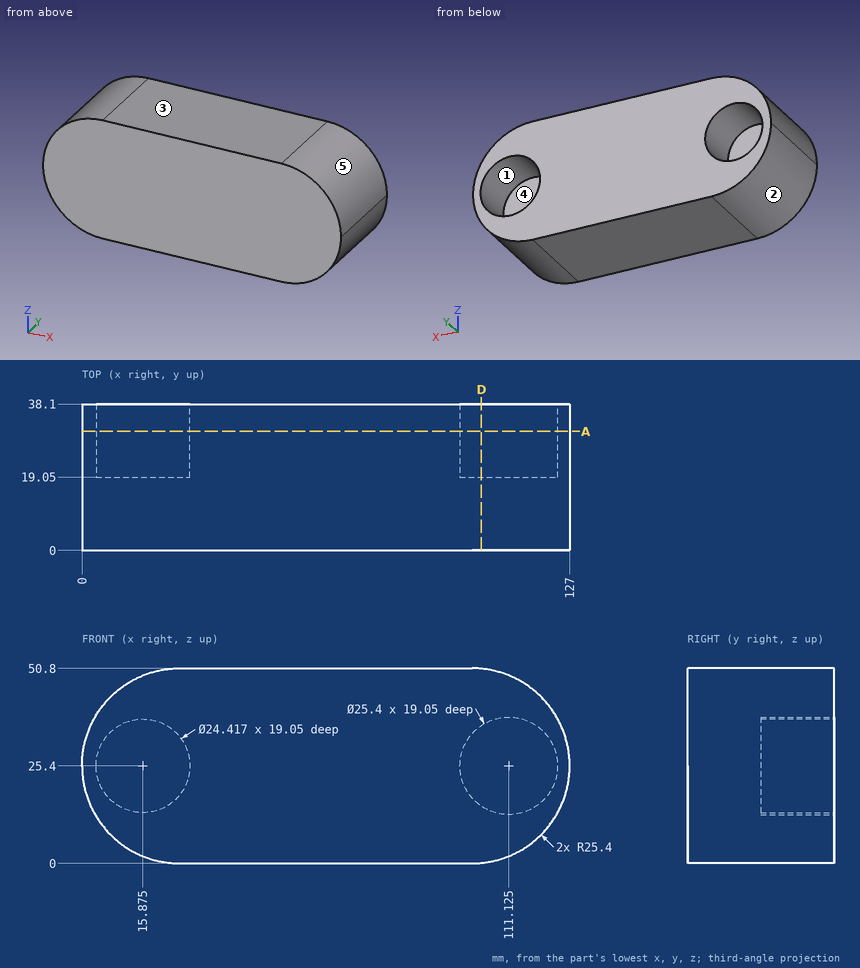
Source: three-view drawing plus pictorial views. Frame: mm from the lowest corner of the part. A direction names the side the tool comes from. Give positions to 0.01 mm unless a question says otherwise; leave off trailing zeros. Write each loop counter-clockwise with the first axis right and the second up, starting at its lowest first coordinate (ties: lowest second). Pieces come first, ordered by that corner, then holes. Notation, with made-up numbers: (12.5, -34.5) - (52.5, -34.5) arc R22 cw to (52.5, -18.5) - close; hole circle Ø3 at (68, -2). An arc over 180 degrees is marked (long way). Write item = value, one per line. Start each with the question number.
1. Section query D-D, the plane x = 104. Output: boundary loops of the cut face in (y, z), then the cut area to 3 significant figures.
2. Section query A-A, the plane y = 31. Count the separate pieces of the cut face and the enclosed holes in it, then the cut area to 3 significant figures.
3. Mould query, pull axis X, two halves, no side actions, for the marked faces 3, 4 and 5. Classes: released by +X, released by -X, zero draft, split by the parting line, or undercut.
4. Access query for the marked faces 1 and 2. Directions: +Z, -Z, +X, -X, +Y, -Y. A direction counts if a zero-diameter tool reaches every point of the face in a straight line with its end or side. Return the directions, or none.
5. First-contact query: pin 1 Ø1.5 at (y, z) = (6.5, 14.5) entering from +X; pin 2 Ø6 at (y, z) = (33, 22) entering from +X; pin 3 Ø12 at (x, z) = (14.5, 24) entering from +Y. Flat tips, straight axial feed; report the tip coordinate or a pass-through.
6. Ray query, L1, parallel to X at y = 24, z = 25; L2, parallel to X at y = 37, z = 28 (1 decimal); L3, parallel to Z at x = 110.5, y = 29 (1 decimal). Return the intervals inside material, ascending.
Check sheet entries:
q1.outline = (0, 0.11) - (38.1, 0.11) - (38.1, 14.89) - (19.05, 14.89) - (19.05, 35.91) - (38.1, 35.91) - (38.1, 50.69) - (0, 50.69) - close
q1.area = 1,530 mm2
q2.separate_pieces = 1
q2.enclosed_holes = 2
q2.area = 4,920 mm2
q3.face_3 = zero draft
q3.face_4 = undercut
q3.face_5 = released by +X
q4.face_1 = +Y
q4.face_2 = -Z, -X, +Y, -Y
q5.pin_1 = 124.88
q5.pin_2 = 127
q5.pin_3 = 19.05
q6.L1 = 0 to 3.67, 28.08 to 98.43, 123.82 to 127
q6.L2 = 0.1 to 3.9, 27.8 to 98.7, 123.6 to 126.9
q6.L3 = 1.6 to 12.7, 38.1 to 49.2
